Work out the finished part from the listing and answer in its coordinate system (mm). Round coordinates to 2 decimals unless told otherwise and drop trailing zeros. Write each loop counter-clockwise with the first axis right and the second up, starting at its lowest first coordinate (ties: lowest second). Pieces come first, ordered by that corner, then holes.
1. Determine the mould class of faces 1 (the face through (3, -86.877, 3)), 2 (the face through (3.31, -59.14, 4.07)), 3 (the face through (11.892, 38, 3)), 4 (the face through (3, 167.123, 3)) for opening direction Y: pulls with the +Y half, pulls with the -Y half, needs draft (parallel to the pull), parting line crosses it, or undercut.
2. Find section A-A (z = 2.25). Write down the section's boundary in (x, y), and give its area (3 significant figures).
3. Straight lines are drawn through the part: probe 1 along Y at (x, z) = (3, 4); probe 2 along Y at (x, z) = (5, 5.5); probe 3 along X at (y, z) = (-8.5, 5). For each, find the intervals that lie inside material, in ascending order.
```python
from build123d import *

# Parameters (mm, degrees)
F0_W           = 17.78
F0_H           = 254
F1_DEPTH       = 6.604
F3_D           = 4.4958
F3_CSINK_D     = 9.1186
F3_CSINK_ANGLE = 82


with BuildPart() as f1:
    # F0 (on Top) → F1 (new body)
    with BuildSketch(Plane.XY):
        with Locations((3.0019969136, 40.122719574)):
            Rectangle(F0_W, F0_H)
    extrude(amount=F1_DEPTH)

    # F3 (through all)
    with Locations(Plane.XY.offset(6.604)):
        with Locations((3.0019969136, 141.722719574), (3.0019969136, 90.922719574), (3.0019969136, 40.122719574), (3.0019969136, -10.677280426), (3.0019969136, -61.477280426)):
            CounterSinkHole(F3_D / 2, F3_CSINK_D / 2, counter_sink_angle=F3_CSINK_ANGLE)


solid = f1.part
```
Worked answers:
1. face 1: pulls with the -Y half
1. face 2: undercut
1. face 3: needs draft
1. face 4: pulls with the +Y half
2. outline: (-5.89, -86.88) - (11.89, -86.88) - (11.89, 167.12) - (-5.89, 167.12) - close; hole circle Ø4.5 at (3, -61.48); hole circle Ø4.5 at (3, -10.68); hole circle Ø4.5 at (3, 40.12); hole circle Ø4.5 at (3, 90.92); hole circle Ø4.5 at (3, 141.72)
2. area: 4,440 mm2
3. probe 1: y = -86.88 to -63.77, -59.18 to -12.97, -8.38 to 37.83, 42.42 to 88.63, 93.22 to 139.43, 144.02 to 167.12
3. probe 2: y = -86.88 to -64.47, -58.48 to -13.67, -7.68 to 37.13, 43.12 to 87.93, 93.92 to 138.73, 144.72 to 167.12
3. probe 3: x = -5.89 to 0.7, 5.3 to 11.89
